Input: part model. Units: mm. Frame: model coordinates. A direction names the side the tool comes from. Give positions to 0.01 mm unless a question says otherwise; leave off trailing zeros. Write each loop counter-clockwise with the first axis right and the second up, starting at its lowest first coordinate (ties: lowest second). Pieces come first, ordered by that corner, then holes. Notation, with made-up numbers: (83.5, 73) - (114.5, 73) arc R13 cw to (114.5, 96) - close; hole circle Ø11 at (53.5, 25). An arc over 180 degrees is marked (long way). Answer as CSV lines item,"result".
```python
from build123d import *

# Parameters (mm, degrees)
SKETCH1_W                 = 25.4
SKETCH1_H                 = 9.525
BOSS_EXTRUDE1_DEPTH       = 80
F_8_32_TAPPED_HOLE1_D     = 3.4544
F_8_32_TAPPED_HOLE1_DEPTH = 19.05
F_8_32_TAPPED_HOLE1_TIP   = 1.037806461
F_8_32_TAPPED_HOLE2_D     = 3.4544
F_8_32_TAPPED_HOLE2_DEPTH = 20.066
F_8_32_TAPPED_HOLE2_TIP   = 1.037806461
F_8_32_TAPPED_HOLE3_D     = 3.4544


with BuildPart() as part:
    # Sketch1 → Boss-Extrude1 (new body)
    with BuildSketch(Plane(origin=(0, 0, 0), x_dir=(1, 0, 0), z_dir=(0, 1, 0))):
        with Locations((-14.638893842, 4.7625)):
            Rectangle(SKETCH1_W, SKETCH1_H)
    extrude(amount=BOSS_EXTRUDE1_DEPTH)

    # #8-32 Tapped Hole1
    with Locations(Plane(origin=(0, 80, 0), x_dir=(1, 0, 0), z_dir=(0, 1, 0))):
        with Locations((-8.288893842, 4.7625), (-20.988893842, 4.7625)):
            Hole(F_8_32_TAPPED_HOLE1_D / 2, depth=F_8_32_TAPPED_HOLE1_DEPTH)
            with Locations((0, 0, -(F_8_32_TAPPED_HOLE1_DEPTH + F_8_32_TAPPED_HOLE1_TIP / 2))):  # 118° drill point
                Cone(0, F_8_32_TAPPED_HOLE1_D / 2, F_8_32_TAPPED_HOLE1_TIP, mode=Mode.SUBTRACT)

    # #8-32 Tapped Hole2
    with Locations(Plane(origin=(0, 0, 0), x_dir=(-1, 0, 0), z_dir=(0, -1, 0))):
        with Locations((20.988893842, 4.7625), (8.288893842, 4.7625)):
            Hole(F_8_32_TAPPED_HOLE2_D / 2, depth=F_8_32_TAPPED_HOLE2_DEPTH)
            with Locations((0, 0, -(F_8_32_TAPPED_HOLE2_DEPTH + F_8_32_TAPPED_HOLE2_TIP / 2))):  # 118° drill point
                Cone(0, F_8_32_TAPPED_HOLE2_D / 2, F_8_32_TAPPED_HOLE2_TIP, mode=Mode.SUBTRACT)

    # #8-32 Tapped Hole3 (through all)
    with Locations(Plane.XY):
        with Locations((-20.988893842, 52.705), (-20.988893842, 27.305)):
            Hole(F_8_32_TAPPED_HOLE3_D / 2)


solid = part.part
```
Item 1: Cut plane A-A on y = 68.5. Return the cut outline in (x, z) (1 decimal), plus the area to 3 significant figures.
The answers:
outline,"(-27.3, -9.5) - (-1.9, -9.5) - (-1.9, 0) - (-27.3, 0) - close; hole circle Ø3.5 at (-21, -4.8); hole circle Ø3.5 at (-8.3, -4.8)"
area,"223 mm²"
Item 2: Reachability of faces 1 (the face through (-10, 10, -5)), 2 (the face through (-22.636, 70.342, -5.281)), 3 (the face through (-15, 0, -5)) from +Z, -Z, +X, -X, +Y, -Y: full face, straight path, thin tool, end or side. Return the list, or none.
The answers:
face 1,"-Y"
face 2,"+Y"
face 3,"+Z, -Z, +X, -X, -Y"
Item 3: Ray query, line 1 (X direction, y = 71, z = -5.5); line 2 (X direction, y = 64, z = -3.75); line 3 (X direction, y = 28, z = -3.5). Return the intervals inside material, ascending. Write a range as from..to.
The answers:
line 1,"-27.34..-22.55, -19.43..-9.85, -6.73..-1.94"
line 2,"-27.34..-22.39, -19.59..-9.69, -6.89..-1.94"
line 3,"-27.34..-22.57, -19.41..-1.94"
Item 4: Mould query, pull axis Z, two halves, no side actions, for faces 4 (the face through (-15, 39, -9.525)), 5 (the face through (-15, 39, 0)), 6 (the face through (-9.217, 70.342, -6.219)). Classes: +Z half, -Z half, draft (parallel to the pull), parting line (faces both ways), or undercut.
The answers:
face 4,"-Z half"
face 5,"+Z half"
face 6,"undercut"
Item 5: Contact query for flat-ended pins moving along their axis: pin 1 (3 mm diameter, centred on x = -20.99, y = 52.7, fed in from -Z); pin 2 (3 mm diameter, centred on x = -8.29, z = -4.76, fed in from -Y); pin 3 (2 mm diameter, centred on x = -20.99, z = -4.76, fed in from -Y). Output: stop coordinate, or through.
The answers:
pin 1,"through"
pin 2,"y = 20.2"
pin 3,"y = 20.5"
